Verification items for the finished model (mm, model axes). A direction names the side the tool comes from. Give positions to 0.01 mm unless a question says otherwise; leave off trailing zeros. Order: outer loops, then holes, each group sorted by start corner. A loop starts at its lowest first (then second) coordinate and runs counter-clockwise, first axis right, second up. Notation, with made-up numbers: (-6.75, 40) - (52.25, 40) arc R19 cw to (52.25, 58) - close; hole circle Ø9 at (76.5, 3). An arc over 180 degrees is marked (long way). Answer as a JSON object with one key per item and string values. Group by question number.
(1) Section check A-A (y = 25). Record the boundary of the cut face in (x, z), then the cut area to 3 significant figures.
(2) Thickness scan on line 1 (Y direction, x = 5, z = -43); line 2 (Z direction, x = 7, y = 40). Record the ranges inside material, lowest first.
(3) Section check D-D (y = 44). Record the boundary of the cut face in (x, z).
(4) Section check B-B (z = 5). Record the boundary of the cut face in (x, y), then the cut area to 4 significant figures.
(5) Access from +Z, -Z, +X, -X, +Y, -Y to the whole of each face (thin tool, end or side, straight path). Record for faces 1 (the face through (-44, 25, 10)), 2 (the face through (7, 25, -45)), 3 (the face through (10, 25, -43)), 4 (the face through (-48, 25, 0)), 5 (the face through (-3, 25, -42)).
(6) Depth check by flat-ended pin: pin 1 Ø1.5 at (y, z) = (32.5, -47) entering from +X; pin 2 Ø2 at (x, y) = (5, 25) entering from -Z; pin 3 Ø21 at (y, z) = (27, 2) entering from +X; pin 4 Ø6 at (x, y) = (-39, 13.5) entering from -Z. Enter the tip coordinate at first touch or a pass-through.
(7) Mould release check, pull along Z, two halves, no side actions. Record for faces 6 (the face through (-32.01, 24.65, -31.63)), 7 (the face through (-43.521, 26.735, 4.772)), 8 (the face through (-33, 50, -31)), 9 (the face through (-34.964, 24.65, -35.742)): +Z half, -Z half, draft (parallel to the pull), parting line (faces both ways), or undercut.
(8) Section check C-C (x = 5). Record the boundary of the cut face in (y, z).
```python
from build123d import *

# Parameters (mm, degrees)
BOSS_EXTRUDE1_DEPTH             = 50
SKETCH2_W                       = 3
SKETCH2_H                       = 50
BOSS_EXTRUDE2_DEPTH             = 10
BOSS_EXTRUDE2_DIRECTION_2_REACH = 88.603
SKETCH4_W                       = 3
SKETCH4_H                       = 50
BOSS_EXTRUDE3_DEPTH             = 10
BOSS_EXTRUDE3_DIRECTION_2_REACH = 88.603
SKETCH5_R                       = 1.75
CUT_EXTRUDE1_DEPTH              = 10
SKETCH6_R                       = 1.75
CUT_EXTRUDE2_DEPTH              = 10


with BuildPart() as part:
    # Sketch1 → Boss-Extrude1 (new body)
    with BuildSketch(Plane(origin=(0, 0, 0), x_dir=(1, 0, 0), z_dir=(0, 1, 0))):
        with BuildLine():
            Line((-50, 0), (-45, 0))
            ThreePointArc((-45, 0), (-31.819805153, 31.819805153), (0, 45))
            Line((0, 45), (0, 50))
            ThreePointArc((0, 50), (-35.355339059, 35.355339059), (-50, 0))
        make_face()
    extrude(amount=BOSS_EXTRUDE1_DEPTH)

    # Sketch2 → Boss-Extrude2 (add)
    with BuildSketch(Plane.XY):
        with Locations((-43.5, 25)):
            Rectangle(SKETCH2_W, SKETCH2_H)
    extrude(amount=BOSS_EXTRUDE2_DEPTH)

    # Sketch2 → Boss-Extrude2 direction 2 (add, up to next)
    with BuildSketch(Plane.XY, mode=Mode.PRIVATE) as boss_extrude2_direction_2_sk1:
        with Locations((-43.5, 25)):
            Rectangle(SKETCH2_W, SKETCH2_H)
    boss_extrude2_direction_2_tool1 = extrude(boss_extrude2_direction_2_sk1.sketch, amount=-BOSS_EXTRUDE2_DIRECTION_2_REACH, mode=Mode.PRIVATE) - part.part
    add(boss_extrude2_direction_2_tool1.solids().sort_by_distance((-43.5, 25, 0))[0])

    # Sketch4 → Boss-Extrude3 (add)
    with BuildSketch(Plane(origin=(0, 0, 0), x_dir=(0, 0, -1), z_dir=(1, 0, 0))):
        with Locations((43.5, 25)):
            Rectangle(SKETCH4_W, SKETCH4_H)
    extrude(amount=BOSS_EXTRUDE3_DEPTH)

    # Sketch4 → Boss-Extrude3 direction 2 (add, up to next)
    with BuildSketch(Plane(origin=(0, 0, 0), x_dir=(0, 0, -1), z_dir=(1, 0, 0)), mode=Mode.PRIVATE) as boss_extrude3_direction_2_sk1:
        with Locations((43.5, 25)):
            Rectangle(SKETCH4_W, SKETCH4_H)
    boss_extrude3_direction_2_tool1 = extrude(boss_extrude3_direction_2_sk1.sketch, amount=-BOSS_EXTRUDE3_DIRECTION_2_REACH, mode=Mode.PRIVATE) - part.part
    add(boss_extrude3_direction_2_tool1.solids().sort_by_distance((0, 25, -43.5))[0])

    # Sketch5 → Cut-Extrude1 (cut)
    with BuildSketch(Plane(origin=(0, 0, -45), x_dir=(-1, 0, 0), z_dir=(0, 0, -1))):
        with Locations((-5, 25)):
            Circle(SKETCH5_R)
    extrude(amount=-CUT_EXTRUDE1_DEPTH, mode=Mode.SUBTRACT)

    # Sketch6 → Cut-Extrude2 (cut)
    with BuildSketch(Plane.ZY.offset(45)):
        with Locations((5, 25)):
            Circle(SKETCH6_R)
    extrude(amount=-CUT_EXTRUDE2_DEPTH, mode=Mode.SUBTRACT)


solid = part.part
```
Solutions:
{
 "1": {"outline": "(-50, 0) arc R50 ccw to (0, -50) - (0, -45) - (3.25, -45) - (3.25, -42) - (-16.16, -42) arc R45 cw to (-42, -16.16) - (-42, 3.25) - (-45, 3.25) - (-45, 0) - close; (-45, 6.75) - (-42, 6.75) - (-42, 10) - (-45, 10) - close; (6.75, -45) - (10, -45) - (10, -42) - (6.75, -42) - close", "area": "477 mm2"},
 "2": {"line 1": "y = 0 to 23.25, 26.75 to 50", "line 2": "z = -45 to -42"},
 "3": {"outline": "(-50, 0) arc R50 ccw to (0, -50) - (0, -45) - (10, -45) - (10, -42) - (-16.16, -42) arc R45 cw to (-42, -16.16) - (-42, 10) - (-45, 10) - (-45, 0) - close"},
 "4": {"outline": "(-45, 0) - (-42, 0) - (-42, 23.25) - (-45, 23.25) - close; (-45, 26.75) - (-42, 26.75) - (-42, 50) - (-45, 50) - close", "area": "139.5 mm2"},
 "5": {"face 1": "+Z, +X, -X, +Y, -Y", "face 2": "-Z, +X, +Y, -Y", "face 3": "+Z, -Z, +X, +Y, -Y", "face 4": "+Z, -X, +Y, -Y", "face 5": "+Z, +X, +Y, -Y"},
 "6": {"pin 1": "stops at x = 0", "pin 2": "passes through", "pin 3": "stops at x = -42", "pin 4": "stops at z = -34.7"},
 "7": {"face 6": "+Z half", "face 7": "undercut", "face 8": "draft", "face 9": "-Z half"},
 "8": {"outline": "(0, -45) - (23.25, -45) - (23.25, -42) - (0, -42) - close; (26.75, -45) - (50, -45) - (50, -42) - (26.75, -42) - close"}
}
